Autodesk Inventor part; units mm, degrees
ref_plane "YZ Plane" through (0, 0, 0) normal (1, 0, 0) x (0, 1, 0)
ref_plane "XZ Plane" through (0, 0, 0) normal (0, 1, 0) x (-1, 0, 0)
ref_plane "XY Plane" through (0, 0, 0) normal (0, 0, 1) x (1, 0, 0)
sketch "Эскиз1" plane through (0, 0, 0) normal (0, 1, 0) x (-1, 0, 0)
  line L0 (0, 0) -> (10.05, 0)
  line L1 (10.05, 0) -> (10.05, -10.05)
  line L2 (10.05, -10.05) -> (0, -10.05)
  line L3 (0, -10.05) -> (0, 0)
  dimension "d0" = 10.05
  dimension "d1" = 10.05
extrude "Выдавливание1" add sketch "Эскиз1" along normal blind 5.6
sketch "Эскиз2" plane through (0, 5.6, 0) normal (0, 1, 0) x (1, 0, 0)
  line L0 (-10.05, 10.05) -> (-10.05, 0)
  line L1 (-10.05, 5.025) -> (0, 5.025)
  line L2 (0, 0) -> (0, 10.05)
  line L3 (-1, 1) -> (-9.05, 1)
  line L4 (-9.05, 1) -> (-9.05, 9.05)
  line L5 (-9.05, 9.05) -> (-1, 9.05)
  line L6 (-1, 9.05) -> (-1, 1)
  line L7 (-1, 1) -> (-9.05, 9.05) construction
  line L8 (-9.05, 1) -> (-1, 9.05) construction
  point P0 (-5.025, 5.025)
  dimension "d4" = 10.05
  dimension "d5" = 10.05
  dimension "d6" = 8.05
  dimension "d7" = 8.05
extrude "Выдавливание2" cut sketch "Эскиз2" against normal blind 1
sketch "Эскиз3" plane through (0, 0, 0) normal (0, -1, 0) x (1, 0, 0)
  line L0 (0, 0) -> (0, -10.05)
  line L1 (0, -5.025) -> (-10.05, -5.025)
  line L2 (-10.05, -10.05) -> (-10.05, 0)
  point P0 (-5.025, -5.025)
hole "Отверстие1" at (-5.025, 0, -5.025) direction (0, 1, 0) diameter 3.2 end through all
sketch "Эскиз4" plane through (0, 0, 0) normal (0, -1, 0) x (1, 0, 0)
  circle A0 centre (-5.025, -5.025) radius 1.6
  line L0 (-6.6416, -7.825) -> (-8.2582, -5.025)
  line L1 (-8.2582, -5.025) -> (-6.6416, -2.225)
  line L2 (-6.6416, -2.225) -> (-3.4084, -2.225)
  line L3 (-3.4084, -2.225) -> (-1.7918, -5.025)
  line L4 (-1.7918, -5.025) -> (-3.4084, -7.825)
  line L5 (-3.4084, -7.825) -> (-6.6416, -7.825)
  point P0 (0, 0)
  dimension "d17" = 5.6
extrude "Выдавливание3" cut sketch "Эскиз4" against normal blind 2.6 contours A0 | L0 L1 L2 L3 L4 L5
properties part number "Тестовая модель (деталь в деталь)"
Can you work these out from the model? Positions are in its coordinate system, mm. A direction names the side the tool comes from. Give positions to 0.01 mm unless a question says otherwise; leave off trailing zeros. Write each loop counter-clockwise with the first axis right and the second up, starting at its lowest first coordinate (ties: lowest second). Pieces come first, ordered by that corner, then holes. Notation, with made-up numbers: (-5.75, 27.25) -> (19.25, 27.25) arc R29 ccw to (19.25, 62.25) -> close; hole circle Ø5 at (61.25, -5). An arc over 180 degrees is marked (long way). Answer as a JSON object with one key per item and string values. Group by question number.
Item 1: Suppose I cut it at B-B (z = -5.5). Please give me the cut outline in (x, y).
Item 2: For faces 4 (the face through (-10.05, 3, -5)), 5 (the face through (-9.05, 5, -5)), 6 (the face through (-2.61, 1.28, -3.61)), which set-ups out of +Z, -Z, +X, -X, +Y, -Y let a thin tool reach every point of the face, with its end or its side?
Item 3: I'm going to push flat-ended pins straight in: P1, Ø4, axis at x = -4, z = -5.5, coming from the +Y side; P2, Ø2.5, axis at x = -5.025, z = -5.025, coming from the +Y side; P3, Ø1.7, axis at x = -6, z = -4.5, coming from the -Y side. Where does each tip first touch, or does it pass through?
Item 4: Suppose I cut it at C-C (x = -6.5). Please give me the cut outline in (y, z) (3 decimals), plus the area to 3 significant figures.
Item 5: Please list where these lines run through material, in increasing order: line 1 (Z direction, x = -4.75, y = 0.8) (3 decimals); line 2 (Z direction, x = -5, y = 3.9). Write a range as [from, to].
Item 6: Suppose I cut it at A-A (y = 5). Please give me the cut outline in (x, z).
Item 7: We'd pull the mould along Z, two halves only. Please class faces 1 (the face through (-5, 5, -1)), 2 (the face through (-0.5, 5.6, -5)), 3 (the face through (-5, 3, 0)): +Z half, -Z half, draft (parallel to the pull), parting line (faces both ways), or undercut.
Item 8: Suppose I cut it at D-D (y = 2.35). Please give me the cut outline in (x, z) (3 decimals), plus the area to 3 significant figures.
Findings:
{
 "1": {"outline": "(-10.05, 0) -> (-7.98, 0) -> (-7.98, 2.6) -> (-6.55, 2.6) -> (-6.55, 4.6) -> (-9.05, 4.6) -> (-9.05, 5.6) -> (-10.05, 5.6) -> close; (-3.5, 2.6) -> (-2.07, 2.6) -> (-2.07, 0) -> (0, 0) -> (0, 5.6) -> (-1, 5.6) -> (-1, 4.6) -> (-3.5, 4.6) -> close"},
 "2": {"face 4": "+Z, -Z, -X, +Y, -Y", "face 5": "+Y", "face 6": "-Y"},
 "3": {"P1": "stops at y = 4.6", "P2": "passes through", "P3": "stops at y = 2.6"},
 "4": {"outline": "(0, -10.05) -> (5.6, -10.05) -> (5.6, -9.05) -> (4.6, -9.05) -> (4.6, -5.645) -> (2.6, -5.645) -> (2.6, -7.825) -> (0, -7.825) -> close; (0, -2.225) -> (2.6, -2.225) -> (2.6, -4.405) -> (4.6, -4.405) -> (4.6, -1) -> (5.6, -1) -> (5.6, 0) -> (0, 0) -> close", "area": "31.2 mm²"},
 "5": {"line 1": "z = [-10.05, -7.825], [-2.225, 0]", "line 2": "z = [-10.05, -6.62], [-3.43, 0]"},
 "6": {"outline": "(-10.05, -10.05) -> (0, -10.05) -> (0, 0) -> (-10.05, 0) -> close; hole (-9.05, -9.05) -> (-1, -9.05) -> (-1, -1) -> (-9.05, -1) -> close"},
 "7": {"face 1": "undercut", "face 2": "draft", "face 3": "+Z half"},
 "8": {"outline": "(-10.05, -10.05) -> (0, -10.05) -> (0, 0) -> (-10.05, 0) -> close; hole (-8.258, -5.025) -> (-6.642, -7.825) -> (-3.408, -7.825) -> (-1.792, -5.025) -> (-3.408, -2.225) -> (-6.642, -2.225) -> close", "area": "73.8 mm²"}
}
